```python
from build123d import *

# Parameters (mm, degrees)
SKETCH1_W           = 344.997499296
SKETCH1_H           = 344.997499295
BOSS_EXTRUDE1_DEPTH = 20
SKETCH2_R           = 3.349999998
CUT_EXTRUDE1_DEPTH  = 21
SKETCH3_W           = 20
SKETCH3_H           = 344.997499295
BOSS_EXTRUDE2_DEPTH = 100


with BuildPart() as part:
    # Sketch1 → Boss-Extrude1 (new body)
    with BuildSketch(Plane.ZY.offset(23098.612597115)):
        with Locations((40779.406254132, 6851.802826482)):
            Rectangle(SKETCH1_W, SKETCH1_H)
    extrude(amount=BOSS_EXTRUDE1_DEPTH)

    # Sketch2 → Cut-Extrude1 (cut, through all)
    with BuildSketch(Plane.ZY.offset(23118.612597115)):
        with Locations((40846.136031778, 6918.532604128)):
            Circle(SKETCH2_R)
        with Locations((40831.993896154, 6904.390468504)):
            Circle(SKETCH2_R)
    extrude(amount=-CUT_EXTRUDE1_DEPTH, mode=Mode.SUBTRACT)

    # Sketch3 → Boss-Extrude2 (add)
    with BuildSketch(Plane.ZY.offset(23118.612597115)):
        with Locations((40616.907504484, 6851.802826482)):
            Rectangle(SKETCH3_W, SKETCH3_H)
    extrude(amount=BOSS_EXTRUDE2_DEPTH)


solid = part.part
```
Can you work these out from the model? Positions are in its coordinate system, mm. A direction names the side the tool comes from. Round coordinates to 2 decimals unless told otherwise and drop trailing zeros. Loops run counter-clockwise (first coordinate to the right, second up) from the corner with the lowest first, then second, coordinate; pieces in that order, holes last. Notation, with made-up numbers: (39.5, -18) -> (66.5, -18) arc R9 ccw to (66.5, -9) -> close; hole circle Ø2 at (-27, 46). An arc over 180 degrees is marked (long way). Answer in a Markdown table with one row per item.
Item 1: On a 3-axis mill with a long thin cutter (end or side, diameter ignored), from which of +Z, -Z, +X, -X, +Y, -Y can I reach the whole of each face in a straight line? I mean faces 1 (the flat face through (-23168, 6849, 40626.908)), 2 (the flat face through (-23118, 7024.302, 40740)). Say none if no direction works.
Answer block:
| item | result |
|---|---|
| face 1 | +Z, -X, +Y, -Y |
| face 2 | +Z, -Z, +X, -X, +Y |
Item 2: Suppose I cut it at A-A, the plane z = 40668. List the corners of the cut face in (x, y) for me, plus the area to 3 significant figures.
Answer block:
| item | result |
|---|---|
| outline | (-23118.61, 6679.3) -> (-23098.61, 6679.3) -> (-23098.61, 7024.3) -> (-23118.61, 7024.3) -> close |
| area | 6,900 mm² |
Item 3: If I drill on probe 1 along X at (y, z) = (6811, 40722); probe 2 along Z at (x, y) = (-23183, 6707), over which ranges is the centre line in solid material (lowest first)?
Answer block:
| item | result |
|---|---|
| probe 1 | -23118.61 to -23098.61 |
| probe 2 | 40606.91 to 40626.91 |
Item 4: Will these pins go through, and if not, where does the flat tip stop? P1, Ø7.5, axis at y = 6918.53, z = 40846.14, coming from the -X side; P2, Ø1, axis at x = -23124, y = 6832.5, coming from the +Z side.
Answer block:
| item | result |
|---|---|
| P1 | x = -23118.61 |
| P2 | z = 40626.91 |
Item 5: Suppose I cut it at C-C, the plane x = -23207.5. List the corners of the cut face in (y, z) for me, plus the area to 3 significant figures.
Answer block:
| item | result |
|---|---|
| outline | (6679.3, 40606.91) -> (7024.3, 40606.91) -> (7024.3, 40626.91) -> (6679.3, 40626.91) -> close |
| area | 6,900 mm² |
Item 6: Suppose I cut it at B-B, the plane y = 6952. List the corners of the cut face in (x, z) for me (1 decimal), plus the area to 3 significant figures.
Answer block:
| item | result |
|---|---|
| outline | (-23218.6, 40606.9) -> (-23098.6, 40606.9) -> (-23098.6, 40951.9) -> (-23118.6, 40951.9) -> (-23118.6, 40626.9) -> (-23218.6, 40626.9) -> close |
| area | 8,900 mm² |
